from build123d import *

# Parameters (mm, degrees)
F0_W      = 12.7
F0_H      = 12.7
F1_DEPTH  = 8.255
F2_R      = 3.0988
F3_DEPTH  = 12.701
F7_R      = 1.016
F8_DEPTH  = 22.89513
F9_R      = 0.25
F10_DEPTH = 24.131


with BuildPart() as f1:
    # F0 (on Top) → F1 (new body)
    with BuildSketch(Plane.XY):
        Rectangle(F0_W, F0_H)
    extrude(amount=F1_DEPTH)

    # F2 (on face) → F3 (cut, through all)
    with BuildSketch(Plane.XZ.offset(6.35)):
        with Locations((2.6924, 4.1275)):
            Circle(F2_R)
    extrude(amount=-F3_DEPTH, mode=Mode.SUBTRACT)

    # F4 (on Front) → F5 (revolve)
    with BuildSketch(Plane.XZ):
        Polygon((-2.3876, 8.255), (-2.3876, 11.43), (-2.9718, 11.43), (-6.35, 9.4996), (-6.35, 8.255), align=None)
    revolve(axis=Axis((-2.3876, 0, 3.00711), (0, 0, -1)))

    # F4 (on Front) → F6 (revolve)
    with BuildSketch(Plane.XZ):
        Polygon((-2.3876, -12.7), (-2.3876, 0), (-6.35, 0), (-6.35, -9.525), (-5.5626, -9.525), (-5.5626, -12.7), align=None)
    revolve(axis=Axis((-2.3876, 0, 3.00711), (0, 0, -1)))

    # F7 (on face) → F8 (cut)
    with BuildSketch(Plane(origin=(0, 0, -12.7), x_dir=(1, 0, 0), z_dir=(0, 0, -1))):
        with Locations((-2.3876, 0)):
            Circle(F7_R)
    extrude(amount=-F8_DEPTH, mode=Mode.SUBTRACT)

    # F9 (on face) → F10 (cut, through all)
    with BuildSketch(Plane.XY.offset(11.43)):
        with Locations((-2.3876, 0)):
            Circle(F9_R)
    extrude(amount=-F10_DEPTH, mode=Mode.SUBTRACT)


solid = f1.part
Build history of the part. All positions in model axes, mm. A direction names the side the tool comes from. Give positions to 0.01 mm unless a question says otherwise; leave off trailing zeros. Write each loop counter-clockwise with the first axis right and the second up, starting at its lowest first coordinate (ties: lowest second). Pieces come first, ordered by that corner, then holes. Notation, with made-up numbers: (47.5, 36) - (94.5, 36) arc R17 ccw to (94.5, 49) - close; hole circle Ø9 at (66.25, -20.5). An arc over 180 degrees is marked (long way). Use one line per item in the form item = value. Start each with the question number.
1. 3-axis set-ups, long thin cutter, end or side, ignore diameter. For faces 4 (the face through (-1.87, 3.93, 8.87)), 5 (the face through (1, 1, -9.525)), 6 (the face through (6.35, 0, 4)): which of +Z, -Z, +X, -X, +Y, -Y reach the whole face in a straight line?
2. Two-plate mould, pull along X, no slides. Class faces 1 (the face through (2.3, -0.1, 7.2)), 2 (the face through (-6.35, 0, 4)), 3 (the face through (-1.87, 3.93, -4.83)): released by +X, released by -X, zero draft, split by the parting line, or undercut.
3. Band-saw the part on B-B on x = 3. Write the cut outline in (y, z) (3 decimals), plus the area to 3 significant figures.
4. Drop flat-ended pins along their axis: pin 1 Ø3 at (x, z) = (2, 3) entering from -Y; pin 2 Ø2 at (x, y) = (3, 0.5) entering from +Z (3 decimals); pin 3 Ø0.6 at (x, y) = (-2, 0) entering from -Z. Give the stop position or say it passes through.
5. Band-saw the part on C-C on z = 2. Write the cut outline in (x, y), plus the area to 3 significant figures.
6. Band-saw the part on A-A on z = 4.5. Write the cut outline in (x, y), plus the area to 3 significant figures.
7. Probe line 1 (Z direction, x = -5.25, y = -3) (3 decimals); line 2 (Z direction, x = 3, y = 5.25) (3 decimals); line 3 (X direction, y = -3.25, z = 5). List the from-to ranges inside material, lowest first. Write a range as [from, to].
Conclusion:
q1.face_4 = +Z
q1.face_5 = -Z
q1.face_6 = +Z, -Z, +X, +Y, -Y
q2.face_1 = undercut
q2.face_2 = released by -X
q2.face_3 = split by the parting line
q3.outline = (-6.35, 0) - (6.35, 0) - (6.35, 1.044) - (-6.35, 1.044) - close; (-6.35, 7.211) - (6.35, 7.211) - (6.35, 8.255) - (-6.35, 8.255) - close
q3.area = 26.5 mm²
q4.pin_1 = through
q4.pin_2 = 8.255
q4.pin_3 = 10.2
q5.outline = (-6.35, -6.35) - (0.44, -6.35) - (0.44, 6.35) - (-6.35, 6.35) - close; (4.95, -6.35) - (6.35, -6.35) - (6.35, 6.35) - (4.95, 6.35) - close; hole circle Ø2.03 at (-2.39, 0)
q5.area = 101 mm²
q6.outline = (-6.35, -6.35) - (-0.38, -6.35) - (-0.38, 6.35) - (-6.35, 6.35) - close; (5.77, -6.35) - (6.35, -6.35) - (6.35, 6.35) - (5.77, 6.35) - close; hole circle Ø2.03 at (-2.39, 0)
q6.area = 79.9 mm²
q7.line_1 = [0, 8.255]
q7.line_2 = [0, 1.044], [7.211, 8.255]
q7.line_3 = [-6.35, -0.28], [5.67, 6.35]
